Part model, mm, in its own coordinate system. A direction names the side the tool comes from. Round coordinates to 2 decimals unless told otherwise and drop trailing zeros. Loops run counter-clockwise (first coordinate to the right, second up) from the corner with the lowest first, then second, coordinate; pieces in that order, holes last. Notation, with made-up numbers: M 66,71.5 L 125,71.5 A22 ccw 125,89.5 Z; hole C 15.25,83 d8. An arc over 180 degrees is marked long. Put each result on its own line as item: value. Start each with the question number.
1) Slice it at A-A on z = 30. Give the cut face in (x, y), then the cut area to 3 significant figures.
2) Slice it at B-B on x = 12. Give the cut face in (y, z), then the cut area to 3 significant figures.
3) Drop flat-ended pins along their axis: pin 1 Ø1.2 at (y, z) = (1.5, 32) entering from +X; pin 2 Ø2 at (y, z) = (57, 198.5) entering from +X; pin 3 Ø2 at (x, y) = (28, 1) entering from +Z. Give the stop position or say it passes through.
4) Slice it at D-D on y = 38.5. Give the cut face in (x, z), then the cut area to 3 significant figures.
5) Which spindle directions (+Z, -Z, +X, -X, +Y, -Y) get a long thin tool onto all of the face, cutting with end or side? Do faces 5 (the flat face through (21, 73.7, 153)), 6 (the flat face through (19, 0, 197)). Say none if no direction does.
6) Probe line 1 along Y through (x, z) = (1.4, 30); line 2 along Y through (x, z) = (0.75, 11.75); line 3 along Y through (x, z) = (15, 257.5). List the from-to ranges inside material, lowest first.
7) Pull direction Y, two halves, no side cores. Call faces 1 (the cylindrical face through (1.232, 57.37, 39.237)), 2 (the flat face through (19, 76.2, 197)), 3 (the flat face through (0, 38, 197)), 4 (the flat face through (2.5, 39, 197)): +Y half, -Y half, draft (parallel to the pull), parting line (faces both ways), or undercut.
8) Slice it at C-C on z = 153. Give the cut face in (x, y), then the cut area to 4 significant figures.
```python
from build123d import *

# Parameters (mm, degrees)
RESSALTO_EXTRUS_O1_DEPTH = 400
ESBO_O3_R                = 10
ESBO_O3_R_2              = 2.5
CORTE_EXTRUS_O1_DEPTH    = 409.971942803
ESBO_O4_W                = 35
ESBO_O4_H                = 60
ESBO_O4_H_2              = 100
CORTE_EXTRUS_O2_DEPTH    = 409.971942803


with BuildPart() as part:
    # Esboço2 → Ressalto-extrusão1 (new body)
    with BuildSketch(Plane.XY):
        Polygon((0, 0), (0, 76.2), (38.1, 76.2), (38.1, 73.7), (2.5, 73.7), (2.5, 2.5), (38.1, 2.5), (38.1, 0), align=None)
    extrude(amount=RESSALTO_EXTRUS_O1_DEPTH)

    # Esboço3 → Corte-extrusão1 (cut, through all)
    with BuildSketch(Plane.ZY):
        with Locations((30, 15)):
            Circle(ESBO_O3_R)
        with Locations((30, 61.2)):
            Circle(ESBO_O3_R)
        with Locations((11.75, 15)):
            Circle(ESBO_O3_R_2)
        with Locations((48.25, 15)):
            Circle(ESBO_O3_R_2)
        with Locations((48.25, 61.2)):
            Circle(ESBO_O3_R_2)
        with Locations((11.75, 61.2)):
            Circle(ESBO_O3_R_2)
    extrude(amount=-CORTE_EXTRUS_O1_DEPTH, mode=Mode.SUBTRACT)

    # Esboço4 → Corte-extrusão2 (cut, through all)
    with BuildSketch(Plane.XZ):
        with Locations((20.6, 30)):
            Rectangle(ESBO_O4_W, ESBO_O4_H)
        with Locations((20.6, 350)):
            Rectangle(ESBO_O4_W, ESBO_O4_H_2)
    extrude(amount=-CORTE_EXTRUS_O2_DEPTH, mode=Mode.SUBTRACT)


solid = part.part
```
Recorded:
1. outline: M 0,0 L 3.1,0 L 3.1,2.5 L 2.5,2.5 L 2.5,5 L 0,5 Z; M 0,25 L 2.5,25 L 2.5,51.2 L 0,51.2 Z; M 0,71.2 L 2.5,71.2 L 2.5,73.7 L 3.1,73.7 L 3.1,76.2 L 0,76.2 Z
1. area: 93.5 mm2
2. outline: M 0,60 L 2.5,60 L 2.5,300 L 0,300 Z; M 73.7,60 L 76.2,60 L 76.2,300 L 73.7,300 Z
2. area: 1,200 mm2
3. pin 1: stops at x = 3.1
3. pin 2: stops at x = 2.5
3. pin 3: stops at z = 300
4. outline: M 0,0 L 2.5,0 L 2.5,400 L 0,400 Z
4. area: 1,000 mm2
5. face 5: +Z, -Z, +X
5. face 6: +Z, -Z, +X, -X, -Y
6. line 1: y = 0 to 5, 25 to 51.2, 71.2 to 76.2
6. line 2: y = 0 to 12.5, 17.5 to 58.7, 63.7 to 76.2
6. line 3: y = 0 to 2.5, 73.7 to 76.2
7. face 1: undercut
7. face 2: +Y half
7. face 3: draft
7. face 4: undercut
8. outline: M 0,0 L 38.1,0 L 38.1,2.5 L 2.5,2.5 L 2.5,73.7 L 38.1,73.7 L 38.1,76.2 L 0,76.2 Z
8. area: 368.5 mm2
